The listing builds one solid part. Answer for the finished solid, in the listing's coordinates (mm). Coordinates: 2 decimals unless noted, no trailing zeros. Write each loop counter-clockwise with the first axis right and the second up, starting at its lowest first coordinate (ties: lowest second). Pieces come first, ordered by that corner, then holes.
from build123d import *

# Parameters (mm, degrees)
F0_R     = 62.5
F0_R_2   = 5
F1_DEPTH = 1


with BuildPart() as f1:
    # F0 (on Front) → F1 (new body, symmetric)
    with BuildSketch(Plane.XZ):
        with BuildLine():
            ThreePointArc((5, 55), (-3.535534, 58.535534), (0, 50))
            ThreePointArc((0, 50), (3.535534, 51.464466), (5, 55))
        make_face()
        with BuildLine():
            ThreePointArc((37.328189, 44.495935), (30.058236, 48.950967), (29.389263, 40.45085))
            ThreePointArc((29.389263, 40.45085), (34.598141, 40.040902), (37.328189, 44.495935))
        make_face()
        Circle(F0_R)
        with Locations((-32.328189, -44.495935)):
            Circle(F0_R_2, mode=Mode.SUBTRACT)
        with Locations((-52.308108, -16.995935)):
            Circle(F0_R_2, mode=Mode.SUBTRACT)
        with Locations((0, -55)):
            Circle(F0_R_2, mode=Mode.SUBTRACT)
        with Locations((32.328189, -44.495935)):
            Circle(F0_R_2, mode=Mode.SUBTRACT)
        with Locations((52.308108, -16.995935)):
            Circle(F0_R_2, mode=Mode.SUBTRACT)
        with Locations((-52.308108, 16.995935)):
            Circle(F0_R_2, mode=Mode.SUBTRACT)
        with Locations((-32.328189, 44.495935)):
            Circle(F0_R_2, mode=Mode.SUBTRACT)
        with BuildLine():
            ThreePointArc((28.434292, 39.136446), (43.102714, 21.96193), (48.375307, 0))
            ThreePointArc((48.375307, 0), (-34.206508, -34.206508), (0, 48.375307))
            ThreePointArc((0, 48.375307), (14.948792, 46.007651), (28.434292, 39.136446))
        make_face(mode=Mode.SUBTRACT)
        with Locations((52.308108, 16.995935)):
            Circle(F0_R_2, mode=Mode.SUBTRACT)
        with BuildLine():
            ThreePointArc((5, 55), (3.535534, 51.464466), (0, 50))
            ThreePointArc((0, 50), (-3.535534, 58.535534), (5, 55))
        make_face(mode=Mode.SUBTRACT)
        with BuildLine():
            ThreePointArc((37.328189, 44.495935), (34.598141, 40.040902), (29.389263, 40.45085))
            ThreePointArc((29.389263, 40.45085), (30.058236, 48.950967), (37.328189, 44.495935))
        make_face(mode=Mode.SUBTRACT)
    extrude(amount=F1_DEPTH, both=True)


solid = f1.part
Q1. The part is cut by section B-B, the plane z = -55. Write down the section's boundary in (x, y).
Answers below:
outline: (-29.69, -1) - (-5, -1) - (-5, 1) - (-29.69, 1) - close; (5, -1) - (29.69, -1) - (29.69, 1) - (5, 1) - close
Q2. Find the intervals of material crossed by probe 1 along Z at (x, y) = (-55.5, 0.25); probe 2 along Z at (x, y) = (-52, 0.35); probe 3 along X at (y, z) = (-0.75, -39), in increasing order.
Answers below:
probe 1: z = -28.74 to -20.84, -13.15 to 13.15, 20.84 to 28.74
probe 2: z = -34.67 to -21.99, -12.01 to 12.01, 21.99 to 34.67
probe 3: x = -48.84 to -28.62, 28.62 to 48.84
Q3. Determine the mould class of faces 1 (the face through (-62.44, -0.01, 2.75)), 2 (the face through (56.927, 0.014, -18.911)), 3 (the face through (-47, -1, 14)) for opening direction Z: released by +Z, released by -Z, zero draft, split by the parting line, or undercut.
Answers below:
face 1: split by the parting line
face 2: undercut
face 3: zero draft
Q4. The part is cut by section C-C, the plane y = 0.05. State how many separate pieces and enclosed holes the cut face has, then the cut area to 3 significant figures.
Answers below:
separate pieces: 1
enclosed holes: 11
area: 4,130 mm2
Q5. The part is cut by section A-A, the plane x = 15. Write down the section's boundary in (y, z), then the cut area to 3 significant figures.
Answers below:
outline: (-1, -60.67) - (1, -60.67) - (1, -45.99) - (-1, -45.99) - close; (-1, 45.99) - (1, 45.99) - (1, 60.67) - (-1, 60.67) - close
area: 58.7 mm2
Q6. The part is cut by section D-D, the plane x = -29. Write down the section's boundary in (y, z), then the cut area to 3 significant figures.
Answers below:
outline: (-1, -55.36) - (1, -55.36) - (1, -48.23) - (-1, -48.23) - close; (-1, -40.76) - (1, -40.76) - (1, -38.72) - (-1, -38.72) - close; (-1, 38.72) - (1, 38.72) - (1, 40.76) - (-1, 40.76) - close; (-1, 48.23) - (1, 48.23) - (1, 55.36) - (-1, 55.36) - close
area: 36.7 mm2
Q7. Given pin 1 (9 mm diameter, centred on x = 32.33, z = -44.5, fed in from -Y); pin 2 (16 mm diameter, centred on x = -32.33, z = -44.5, fed in from -Y), each flat-ended and moving along its own axis, determine where each tip first touches the part or whether it passes through.
Answers below:
pin 1: passes through
pin 2: stops at y = -1
